For this review, take the finished solid that the model builds, in its own axes (mm). Face numbers are marked on the shaded views. A direction names the side the tool comes from. Round coordinates to 2 decimals unless told otherwise and drop trailing zeros. Order: outer loops, then holes, each group sorted by start corner. A loop starts at its lowest first (then second) coordinate and runs counter-clockwise, first axis right, second up. Notation, with made-up numbers: M -11,25.25 L 15,25.25 A21 cw 15,37.25 Z; hole C 56.5,89.25 d6. An arc over 180 degrees is marked long. Use a Markdown table: item, result.
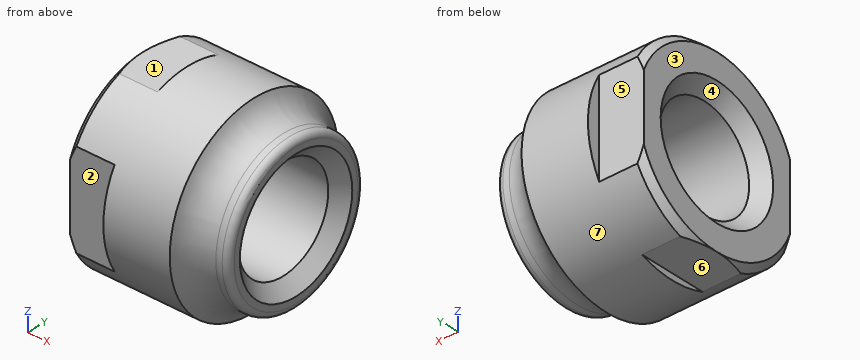
from build123d import *

# Parameters (mm, degrees)
CONG_1_R                = 0.5
CHANFREIN1_SIZE         = 1
CHANFREIN2_SIZE         = 0.5
ESQUISSE2_OUTSIDE_W     = 21.874
ESQUISSE2_OUTSIDE_H     = 21.874
ESQUISSE2_OUTSIDE_W_2   = 14
ESQUISSE2_OUTSIDE_H_2   = 13
ENL_V_MAT_EXTRU_1_DEPTH = 3.5


with BuildPart() as part:
    # Esquisse1 → Révolution1 (revolve)
    with BuildSketch(Plane.XY, mode=Mode.PRIVATE) as r_volution1_sk:
        with BuildLine():
            Line((0, 6), (1, 6))
            Line((1, 6), (1, 4))
            Line((1, 4), (-11, 4))
            Line((-11, 4), (-11, 7.5))
            Line((-11, 7.5), (-2.291287847, 7.5))
            ThreePointArc((-2.291287847, 7.5), (-1.369306394, 6.408349934), (0, 6))
        make_face()
    revolve(r_volution1_sk.sketch.rotate(Axis((-14.539906675, 0, 0), (1, 0, 0)), 90), axis=Axis((-14.539906675, 0, 0), (1, 0, 0)))  # turned: the seam where the file's is

    # Congé1
    cong_1_edges = [part.edges().sort_by_distance(p)[0] for p in [
        (1, 0, -6),
    ]]
    fillet(cong_1_edges, radius=CONG_1_R)

    # Chanfrein1
    chanfrein1_edges = [part.edges().sort_by_distance(p)[0] for p in [
        (1, 0, -4),
        (-11, 0, -4),
    ]]
    chamfer(chanfrein1_edges, length=CHANFREIN1_SIZE)

    # Chanfrein2
    chanfrein2_edges = [part.edges().sort_by_distance(p)[0] for p in [
        (-11, 0, -7.5),
    ]]
    chamfer(chanfrein2_edges, length=CHANFREIN2_SIZE)

    # Esquisse2 outside → Enlèv. mat.-Extru.1 (cut)
    with BuildSketch(Plane.ZY.offset(11)):
        Rectangle(ESQUISSE2_OUTSIDE_W, ESQUISSE2_OUTSIDE_H)
        Rectangle(ESQUISSE2_OUTSIDE_W_2, ESQUISSE2_OUTSIDE_H_2, mode=Mode.SUBTRACT)
    extrude(amount=-ENL_V_MAT_EXTRU_1_DEPTH, mode=Mode.SUBTRACT)


solid = part.part
Q1. Machinability: for the marked faces 1, 2 and 3, which of the approach directions +Z, -Z, +X, -X, +Y, -Y give a long, thin tool a straight path to every point of the face, cutting with its end or side? Answer none if there is none.
Determined:
| item | result |
|---|---|
| face 1 | +Z, -X, +Y, -Y |
| face 2 | +Z, -Z, -X, -Y |
| face 3 | +Z, -Z, -X, +Y, -Y |
Q2. Add section A-A (z = 0). Write out the cut boundary in (x, y), then the cut area to 3 significant figures.
Determined:
| item | result |
|---|---|
| outline | M -11,-6.5 L -7.5,-6.5 L -7.5,-7.5 L -2.29,-7.5 A2.5 cw 0,-6 L 0.5,-6 A0.5 ccw 1,-5.5 L 1,-5 L 0,-4 L -10,-4 L -11,-5 Z; M -11,5 L -10,4 L 0,4 L 1,5 L 1,5.5 A0.5 ccw 0.5,6 L 0,6 A2.5 cw -2.29,7.5 L -7.5,7.5 L -7.5,6.5 L -11,6.5 Z |
| area | 66.9 mm^2 |
Q3. Draft analysis for pull direction Z (two halves, no side actions). For the marked faces 4, 5, 6 and 7, state which applies: pulls with the +Z half, pulls with the -Z half, needs draft (parallel to the pull), parting line crosses it, or undercut.
Determined:
| item | result |
|---|---|
| face 4 | undercut |
| face 5 | needs draft |
| face 6 | pulls with the -Z half |
| face 7 | parting line crosses it |
Q4. Add section B-B (x = -4). Write out the cut boundary in (y, z).
Determined:
| item | result |
|---|---|
| outline | C 0,0 d15; hole C 0,0 d8 |
Q5. Wall thickness on line 1 along Y through (x, z) = (-6.5, 0); line 2 along Z through (x, y) = (-8.75, 0.25); line 3 along Y through (x, z) = (-6.75, -1): over which ranges is each line inside the solid? List them lowest first. Write a range as [from, to].
Determined:
| item | result |
|---|---|
| line 1 | y = [-7.5, -4], [4, 7.5] |
| line 2 | z = [-7, -3.99], [3.99, 7] |
| line 3 | y = [-7.43, -3.87], [3.87, 7.43] |
Q6. Clearance check with flat-ended pins moving along their axes: pin 1 (3 mm diameter, centred on x = -9.5, z = 1.5, fed in from -Y); pin 2 (2 mm diameter, centred on x = -3.5, z = -3, fed in from +Y); pin 3 (5 mm diameter, centred on x = -2.5, y = -5, fed in from +Z); pin 4 (1.1 mm diameter, centred on y = 7, z = 0, fed in from -X). State where each tip first meets the part, or that it passes through.
Determined:
| item | result |
|---|---|
| pin 1 | stops at y = -6.5 |
| pin 2 | stops at y = 7.23 |
| pin 3 | stops at z = 7.07 |
| pin 4 | stops at x = -11 |
